Build history of the part. All positions in model axes, mm. Face numbers are marked on the shaded views. A direction names the side the tool comes from. Round coordinates to 2 decimals unless told otherwise and drop trailing zeros. Write each loop counter-clockwise with the first axis right and the second up, starting at its lowest first coordinate (ties: lowest second). Pieces come first, ordered by that corner, then holes. Notation, with made-up numbers: M 29.5,29 L 68.5,29 A21 cw 68.5,65 Z; hole C 6.5,-39 d9. An arc over 180 degrees is marked long. Use a Markdown table: item, result.
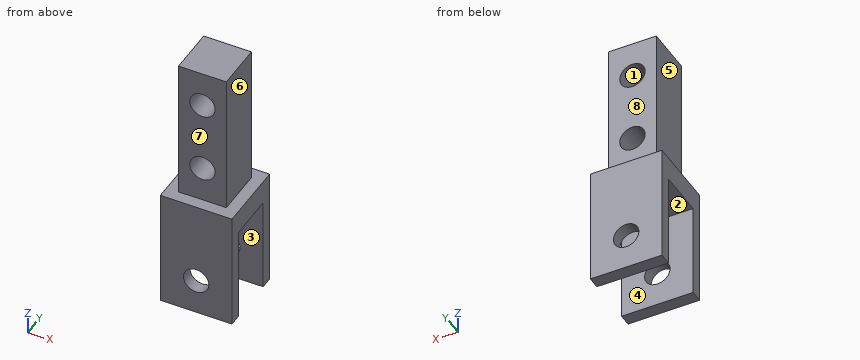
from build123d import *

# Parameters (mm, degrees)
SKETCH1_W                   = 12.7
SKETCH1_H                   = 12.7
BOSS_EXTRUDE1_DEPTH         = 38.1
SKETCH2_W                   = 19.05
SKETCH2_H                   = 19.05
BOSS_EXTRUDE2_DEPTH         = 31.75
SKETCH3_W                   = 25.4
SKETCH3_H                   = 12.446
CUT_EXTRUDE1_DEPTH          = 44.649033494
F_1_4_CLEARANCE_HOLE1_D     = 6.7564
F_1_4_CLEARANCE_HOLE1_DEPTH = 19.05
F_1_4_CLEARANCE_HOLE1_TIP   = 2.029827343


with BuildPart() as part:
    # Sketch1 → Boss-Extrude1 (new body)
    with BuildSketch(Plane.XY):
        Rectangle(SKETCH1_W, SKETCH1_H)
    extrude(amount=BOSS_EXTRUDE1_DEPTH)

    # Sketch2 → Boss-Extrude2 (add)
    with BuildSketch(Plane.XY):
        Rectangle(SKETCH2_W, SKETCH2_H)
    extrude(amount=-BOSS_EXTRUDE2_DEPTH)

    # Sketch3 → Cut-Extrude1 (cut, through all)
    with BuildSketch(Plane.ZY.offset(9.525)):
        with Locations((-19.05, 0)):
            Rectangle(SKETCH3_W, SKETCH3_H)
    extrude(amount=-CUT_EXTRUDE1_DEPTH, mode=Mode.SUBTRACT)

    # 1/4 Clearance Hole1
    with Locations(Plane(origin=(47.625, 9.525, -52.822499938), x_dir=(0, 0, 1), z_dir=(0, 1, 0))):
        with Locations((30.597499938, -47.625), (62.347499938, -47.625), (81.397499938, -47.625), (196.332499938, -47.625)):
            Hole(F_1_4_CLEARANCE_HOLE1_D / 2, depth=F_1_4_CLEARANCE_HOLE1_DEPTH)
            with Locations((0, 0, -(F_1_4_CLEARANCE_HOLE1_DEPTH + F_1_4_CLEARANCE_HOLE1_TIP / 2))):  # 118° drill point
                Cone(0, F_1_4_CLEARANCE_HOLE1_D / 2, F_1_4_CLEARANCE_HOLE1_TIP, mode=Mode.SUBTRACT)


solid = part.part
Q1. Cut at A-A on x = 0. Give the cut face in (y, z) (3 decimals), and give its area (3 significant figures).
Response values:
| item | result |
|---|---|
| outline | M -9.525,-31.75 L -6.223,-31.75 L -6.223,-25.603 L -9.525,-25.603 Z; M -9.525,-18.847 L -6.223,-18.847 L -6.223,-6.35 L 6.223,-6.35 L 6.223,-18.847 L 9.525,-18.847 L 9.525,0 L 6.35,0 L 6.35,6.147 L -6.35,6.147 L -6.35,0 L -9.525,0 Z; M -6.35,12.903 L 6.35,12.903 L 6.35,25.197 L -6.35,25.197 Z; M -6.35,31.953 L 6.35,31.953 L 6.35,38.1 L -6.35,38.1 Z; M 6.223,-31.75 L 9.525,-31.75 L 9.525,-25.603 L 6.223,-25.603 Z |
| area | 556 mm2 |
Q2. Cut at C-C on z = -16.5. Give the cut face in (x, y) (3 decimals).
Response values:
| item | result |
|---|---|
| outline | M -9.525,-9.525 L 9.525,-9.525 L 9.525,-6.223 L -9.525,-6.223 Z; M -9.525,6.223 L 9.525,6.223 L 9.525,9.525 L -9.525,9.525 Z |
Q3. Cut at B-B on y = -3.75. Give the cut face in (x, z) (3 decimals), and give its area (3 significant figures).
Response values:
| item | result |
|---|---|
| outline | M -9.525,-6.35 L 9.525,-6.35 L 9.525,0 L 6.35,0 L 6.35,38.1 L -6.35,38.1 L -6.35,0 L -9.525,0 Z; hole C 0,9.525 d6.756; hole C 0,28.575 d6.756 |
| area | 533 mm2 |
Q4. Drop flat-ended pins along their axis: P1, Ø11, axis at x = 0, z = -22.225, coming from the +Y side (3 decimals); P2, Ø4, axis at x = 0, z = 24.5, coming from the +Y side; P3, Ø10, axis at y = -2.5, z = 19, coming from the -X side; P4, Ø10, axis at y = 2.5, z = 11, coming from the +X side. Give the stop position or say it passes through.
Response values:
| item | result |
|---|---|
| P1 | stops at y = 9.525 |
| P2 | stops at y = 6.35 |
| P3 | stops at x = -6.35 |
| P4 | stops at x = 6.35 |
Q5. Cut at D-D on x = -4.5. Give the cut face in (y, z) (3 decimals), and give its area (3 significant figures).
Response values:
| item | result |
|---|---|
| outline | M -9.525,-31.75 L -6.223,-31.75 L -6.223,-6.35 L 6.223,-6.35 L 6.223,-31.75 L 9.525,-31.75 L 9.525,0 L 6.35,0 L 6.35,38.1 L -6.35,38.1 L -6.35,0 L -9.525,0 Z |
| area | 773 mm2 |
Q6. Which spindle directions (+Z, -Z, +X, -X, +Y, -Y) get a long thin tool onto all of the face, cutting with end or side? Do the marked faces 4, 5, 6, 7 and 8. Say none if no direction does.
Response values:
| item | result |
|---|---|
| face 4 | -Z, +X, -X |
| face 5 | +Z, -X, +Y, -Y |
| face 6 | +Z, +X, +Y, -Y |
| face 7 | +Z, +X, -X, -Y |
| face 8 | +Z, +X, -X, +Y |
Q7. Two-plate mould, pull along Z, no slides. Class the marked faces 1, 2 and 3: +Z half, -Z half, draft (parallel to the pull), parting line (faces both ways), or undercut.
Response values:
| item | result |
|---|---|
| face 1 | undercut |
| face 2 | -Z half |
| face 3 | draft |
Q8. Drill centre lines: L1, parallel to Y at x = 3, z = -14 (3 decimals); L2, parallel to Z at x = -0.5, y = -5; L3, parallel to Z at x = -1, y = 5. Where is each one in solid material? Low to high.
Response values:
| item | result |
|---|---|
| L1 | y = -9.525 to -6.223, 6.223 to 9.525 |
| L2 | z = -6.35 to 6.18, 12.87 to 25.23, 31.92 to 38.1 |
| L3 | z = -6.35 to 6.3, 12.75 to 25.35, 31.8 to 38.1 |
